Could you check a few things on this model? Use its own coordinates, in mm. A direction names the side the tool comes from. Coordinates: 2 decimals unless noted, no trailing zeros. Loops run counter-clockwise (first coordinate to the right, second up) from the corner with the lowest first, then second, coordinate; pieces in that order, holes last.
1) Imagine slicing it at B-B on x = 63. Please give me the cut outline in (y, z), plus the area to 3 significant figures.
2) Thinking about a two-plate mould opening in Y: for faces 1 (the face through (57, 19, 3)), 2 (the face through (47, 65, 1)), 3 (the face through (47, 0, 1)), which applies, released by +Y, released by -Y, zero draft, split by the parting line, or undercut?
3) If I drill on line 1 along Y through (x, z) = (12, 1.4); line 2 along Y through (x, z) = (63, 1.2); line 3 along Y through (x, z) = (8, 0.5), over which ranges is the centre line in solid material (lowest first)?
4) For faces 4 (the face through (95, 32, 1)), 5 (the face through (94, 32, 1)), 6 (the face through (91, 6, 2.3)), which set-ups out of +Z, -Z, +X, -X, +Y, -Y let a thin tool reach every point of the face, with its end or its side?
5) Imagine slicing it at C-C on x = 12. Give the number of separate pieces and of enclosed holes in the cut face, plus the area to 3 significant figures.
6) Will these pins go through, and if not, where does the flat tip stop? P1, Ø4.5, axis at x = 63, y = 59.5, coming from the +Z side; P2, Ø1, axis at y = 47, z = 4.5, coming from the -X side; P3, Ø2, axis at x = 89, y = 4.5, coming from the +Z side; P4, Ø12, axis at x = 65, y = 26.5, coming from the -Z side.
7) Imagine slicing it at A-A on y = 24.5. Please give me the cut outline in (x, z), plus the area to 3 significant figures.
```python
from build123d import *

# Parameters (mm, degrees)
EXTRUDE_346_DEPTH           = 5
EXTRUDE_346_DEPTH_BACK      = 1.1
SKETCH_2_W                  = 95
SKETCH_2_H                  = 65
SKETCH_3_W                  = 56
SKETCH_3_H                  = 38.5
CUT_EXTRUDE_448_DEPTH       = 5
CUT_EXTRUDE_527_DEPTH       = 3
CUT_EXTRUDE_527_DEPTH_BACK  = 1.1
SKETCH_4_W                  = 93
SKETCH_4_H                  = 63
CUT_EXTRUDE_START           = 5
SKETCH_5_W                  = 91
SKETCH_5_H                  = 61
CUT_EXTRUDE_612_DEPTH       = 1
CUT_EXTRUDE_START_2         = 4
SKETCH_6_W                  = 16
SKETCH_6_H                  = 3
CUT_EXTRUDE_697_DEPTH       = 1
WRAP_1_OUTLINE_R            = 3
WRAP_1_DEPTH                = 2.6
SKETCH_13_R                 = 1.1
CUT_EXTRUDE_1_DEPTH         = 116.221569161
SKETCH_15_R                 = 3
EXTRUDE_2_DEPTH             = 2.6
OTHER_START                 = 0.4
OTHER_2_OUTLINE_R           = 1.1
OTHER_2_DEPTH               = 3.6
SKETCH_16_R                 = 3
EXTRUDE_3_DEPTH             = 2.6
OTHER_3_OUTLINE_R           = 1.1
OTHER_3_DEPTH               = 3.6
EXTRUDE_1_DEPTH             = 4.1
EXTRUDE_2_2_DEPTH           = 4.1
EXTRUDE_3_2_DEPTH           = 4.1
EXTRUDE_4_DEPTH             = 4.1
CUT_EXTRUDE_3053_DEPTH      = 0.4
CUT_EXTRUDE_3053_DEPTH_BACK = 1.1
SKETCH_21_W                 = 91.4
SKETCH_21_H                 = 61.4
CUT_EXTRUDE_1_2_DEPTH       = 1.7
CUT_EXTRUDE_2_DEPTH         = 1.7
CUT_EXTRUDE_3_DEPTH         = 1.7
FILLET_1_R                  = 1
FILLET_2_R                  = 1
FILLET_3_R                  = 1
FILLET_4_R                  = 1


# Read off the part's stored shape, not the designer's step: Стойка1, Отверстие2, Отверстие3
with BuildPart() as part:
    # Эскиз2 → Extrude 346 (new, two sides: drawn at the far end of the back side and taken through both)
    with BuildSketch(Plane.XY.offset(-EXTRUDE_346_DEPTH_BACK)):
        with Locations((47.5, 32.5)):
            Rectangle(SKETCH_2_W, SKETCH_2_H)
    extrude(amount=EXTRUDE_346_DEPTH + EXTRUDE_346_DEPTH_BACK)

    # Эскиз3 → Cut-Extrude 448 (cut)
    with BuildSketch(Plane.XY):
        with Locations((32, 40.75)):
            Rectangle(SKETCH_3_W, SKETCH_3_H)
    extrude(amount=CUT_EXTRUDE_448_DEPTH, mode=Mode.SUBTRACT)

    # Эскиз4 → Cut-Extrude 527 (cut, two sides: drawn at the far end of the back side and taken through both)
    with BuildSketch(Plane.XY.offset(-CUT_EXTRUDE_527_DEPTH_BACK)):
        with Locations((47.5, 32.5)):
            Rectangle(SKETCH_4_W, SKETCH_4_H)
    extrude(amount=CUT_EXTRUDE_527_DEPTH + CUT_EXTRUDE_527_DEPTH_BACK, mode=Mode.SUBTRACT)

    # Эскиз5 → Cut-Extrude 612 (cut)
    with BuildSketch(Plane.XY.offset(CUT_EXTRUDE_START)):
        with Locations((47.5, 32.5)):
            Rectangle(SKETCH_5_W, SKETCH_5_H)
    extrude(amount=-CUT_EXTRUDE_612_DEPTH, mode=Mode.SUBTRACT)

    # Эскиз6 → Cut-Extrude 697 (cut)
    with BuildSketch(Plane.XY.offset(CUT_EXTRUDE_START_2)):
        with Locations((78.5, 5.5)):
            Rectangle(SKETCH_6_W, SKETCH_6_H)
    extrude(amount=-CUT_EXTRUDE_697_DEPTH, mode=Mode.SUBTRACT)

    # Стойка1 outline → Стойка1 (add)
    with BuildSketch(Plane(origin=(0, 0, 3), x_dir=(-1, 0, 0), z_dir=(0, 0, -1))):
        with Locations((-12, 17)):
            Circle(WRAP_1_OUTLINE_R)
    extrude(amount=WRAP_1_DEPTH)

    # Эскиз13 → Cut-Extrude 1 (cut, through all)
    with BuildSketch(Plane.XY.offset(4)):
        with Locations((12, 17)):
            Circle(SKETCH_13_R)
    extrude(amount=-CUT_EXTRUDE_1_DEPTH, mode=Mode.SUBTRACT)

    # Эскиз15 → Extrude 2 (add)
    with BuildSketch(Plane(origin=(0, 0, 3), x_dir=(-1, 0, 0), z_dir=(0, 0, -1))):
        with Locations((-63, 59.5)):
            Circle(SKETCH_15_R)
    extrude(amount=EXTRUDE_2_DEPTH)

    # Отверстие2 outline → Отверстие2 (cut)
    with BuildSketch(Plane.XY.offset(OTHER_START)):
        with Locations((63, 59.5)):
            Circle(OTHER_2_OUTLINE_R)
    extrude(amount=OTHER_2_DEPTH, mode=Mode.SUBTRACT)

    # Эскиз16 → Extrude 3 (add)
    with BuildSketch(Plane(origin=(0, 0, 3), x_dir=(-1, 0, 0), z_dir=(0, 0, -1))):
        with Locations((-89.5, 5.5)):
            Circle(SKETCH_16_R)
    extrude(amount=EXTRUDE_3_DEPTH)

    # Отверстие3 outline → Отверстие3 (cut)
    with BuildSketch(Plane.XY.offset(OTHER_START)):
        with Locations((89.5, 5.5)):
            Circle(OTHER_3_OUTLINE_R)
    extrude(amount=OTHER_3_DEPTH, mode=Mode.SUBTRACT)

    # Эскиз22 → Угол1 (add)
    with BuildSketch(Plane(origin=(0, 0, 3), x_dir=(-1, 0, 0), z_dir=(0, 0, -1))):
        Polygon((-1, 64), (-1, 60), (-5, 64), align=None)
    extrude(amount=EXTRUDE_1_DEPTH)

    # Эскиз20 → Extrude 2 2 (add)
    with BuildSketch(Plane(origin=(0, 0, 3), x_dir=(-1, 0, 0), z_dir=(0, 0, -1))):
        Polygon((-1, 1), (-1, 5), (-5, 1), align=None)
    extrude(amount=EXTRUDE_2_2_DEPTH)

    # Эскиз23 → Extrude 3 2 (add)
    with BuildSketch(Plane(origin=(0, 0, 3), x_dir=(-1, 0, 0), z_dir=(0, 0, -1))):
        Polygon((-94, 1), (-90, 1), (-94, 5), align=None)
    extrude(amount=EXTRUDE_3_2_DEPTH)

    # Эскиз24 → Угол4 (add)
    with BuildSketch(Plane(origin=(0, 0, 3), x_dir=(-1, 0, 0), z_dir=(0, 0, -1))):
        Polygon((-94, 64), (-90, 64), (-94, 60), align=None)
    extrude(amount=EXTRUDE_4_DEPTH)

    # Эскиз21 → Cut-Extrude 3053 (cut, two sides: drawn at the far end of the back side and taken through both)
    with BuildSketch(Plane.XY.offset(-CUT_EXTRUDE_3053_DEPTH_BACK)):
        with Locations((47.5, 32.5)):
            Rectangle(SKETCH_21_W, SKETCH_21_H)
    extrude(amount=CUT_EXTRUDE_3053_DEPTH + CUT_EXTRUDE_3053_DEPTH_BACK, mode=Mode.SUBTRACT)

    # Эскиз25 → Cut-Extrude 1 2 (cut)
    with BuildSketch(Plane.XY.offset(4)):
        Polygon((9.632863896, 17), (10.816431948, 14.95), (13.183568052, 14.95), (14.367136104, 17), (13.183568052, 19.05), (10.816431948, 19.05), align=None)
    extrude(amount=-CUT_EXTRUDE_1_2_DEPTH, mode=Mode.SUBTRACT)

    # Эскиз27 → Гайка2 (cut)
    with BuildSketch(Plane.XY.offset(4)):
        Polygon((65.367136104, 59.5), (64.183568052, 61.55), (61.816431948, 61.55), (60.632863896, 59.5), (61.816431948, 57.45), (64.183568052, 57.45), align=None)
    extrude(amount=-CUT_EXTRUDE_2_DEPTH, mode=Mode.SUBTRACT)

    # Эскиз28 → Гайка3 (cut)
    with BuildSketch(Plane.XY.offset(4)):
        Polygon((91.867136104, 5.5), (90.683568052, 7.55), (88.316431948, 7.55), (87.132863896, 5.5), (88.316431948, 3.45), (90.683568052, 3.45), align=None)
    extrude(amount=-CUT_EXTRUDE_3_DEPTH, mode=Mode.SUBTRACT)

    # Скругление1
    fillet_1_edges = [part.edges().sort_by_distance(p)[0] for p in [
        (47.5, 65, 5),
    ]]
    fillet(fillet_1_edges, radius=FILLET_1_R)

    # Скругление2
    fillet_2_edges = [part.edges().sort_by_distance(p)[0] for p in [
        (95, 32, 5),
        (95, 64.707106781, 4.707106781),
        (95, 65, 1.45),
    ]]
    fillet(fillet_2_edges, radius=FILLET_2_R)

    # Скругление3
    fillet_3_edges = [part.edges().sort_by_distance(p)[0] for p in [
        (47, 0, 5),
        (94.707106781, 0, 4.707106781),
        (95, 0, 1.45),
    ]]
    fillet(fillet_3_edges, radius=FILLET_3_R)

    # Скругление4
    fillet_4_edges = [part.edges().sort_by_distance(p)[0] for p in [
        (0, 32.5, 5),
        (0, 64.707106781, 4.707106781),
        (0, 0.292893219, 4.707106781),
        (0, 65, 1.45),
        (0, 0, 1.45),
    ]]
    fillet(fillet_4_edges, radius=FILLET_4_R)


solid = part.part
```
Filled in:
1. outline: (0, -1.1) - (1, -1.1) - (1, 3) - (56.5, 3) - (56.5, 0.4) - (58.4, 0.4) - (58.4, 2.3) - (57.45, 2.3) - (57.45, 4) - (2, 4) - (2, 5) - (1, 5) arc R1 ccw to (0, 4) - close; (60.6, 0.4) - (62.5, 0.4) - (62.5, 3) - (64, 3) - (64, -1.1) - (65, -1.1) - (65, 4) arc R1 ccw to (64, 5) - (63, 5) - (63, 4) - (61.55, 4) - (61.55, 2.3) - (60.6, 2.3) - close
1. area: 81.2 mm2
2. face 1: undercut
2. face 2: released by +Y
2. face 3: released by -Y
3. line 1: y = 0 to 1, 14 to 15.9, 18.1 to 20, 64 to 65
3. line 2: y = 0 to 1, 56.5 to 58.4, 60.6 to 62.5, 64 to 65
3. line 3: y = 0 to 1, 64 to 65
4. face 4: +Z, -Z, +X, +Y, -Y
4. face 5: -Z
4. face 6: +Z
5. separate pieces: 3
5. enclosed holes: 0
5. area: 42.7 mm2
6. P1: stops at z = 4
6. P2: stops at x = 0
6. P3: stops at z = 2.3
6. P4: stops at z = 3
7. outline: (0, -1.1) - (1, -1.1) - (1, 3) - (4, 3) - (4, 4) - (2, 4) - (2, 5) - (1, 5) arc R1 ccw to (0, 4) - close; (60, 3) - (94, 3) - (94, -1.1) - (95, -1.1) - (95, 4) arc R1 ccw to (94, 5) - (93, 5) - (93, 4) - (60, 4) - close
7. area: 50.8 mm2
